```python
from build123d import *

# Parameters (mm, degrees)
BOSS_EXTRUDE3_DEPTH = 23
SKETCH5_W           = 86
SKETCH5_H           = 89
BOSS_EXTRUDE4_DEPTH = 4
SKETCH7_W           = 86
SKETCH7_H           = 4
CUT_EXTRUDE2_DEPTH  = 6
FILLET2_R           = 2
FILLET3_R           = 2
SKETCH8_R           = 1.6
BOSS_EXTRUDE5_DEPTH = 4
FILLET4_R           = 2


# Some blends are built 0.0001 mm under size
with BuildPart() as part:
    # Sketch2 → Boss-Extrude3 (new body)
    with BuildSketch(Plane(origin=(0, 0, 0), x_dir=(1, 0, 0), z_dir=(0, 1, 0))):
        Polygon((-45.956172868, 28.642659602), (-45.956172868, -110.357340398), (40.043827132, -110.357340398), (40.043827132, 28.642659602), (36.043827132, 28.642659602), (36.043827132, -106.357340398), (-41.956172868, -106.357340398), (-41.956172868, 28.642659602), align=None)
    extrude(amount=BOSS_EXTRUDE3_DEPTH)

    # Sketch5 → Boss-Extrude4 (add)
    with BuildSketch(Plane.XZ):
        with Locations((-2.956172868, 65.857340398)):
            Rectangle(SKETCH5_W, SKETCH5_H)
    extrude(amount=BOSS_EXTRUDE4_DEPTH)

    # Sketch7 → Cut-Extrude2 (cut)
    with BuildSketch(Plane.XZ):
        with Locations((-2.956172868, -20.642659602)):
            Rectangle(SKETCH7_W, SKETCH7_H)
    extrude(amount=-CUT_EXTRUDE2_DEPTH, mode=Mode.SUBTRACT)

    # Fillet2
    fillet2_edges = [part.edges().sort_by_distance(p)[0] for p in [
        (40.043827132, -4, 65.857340398),
        (-2.956172868, -4, 110.357340398),
        (-45.956172868, -4, 65.857340398),
    ]]
    fillet(fillet2_edges, radius=FILLET2_R)

    # Fillet3
    # the kernel refuses this fillet: 2 mm, written as the material it takes off along each edge
    with BuildSketch(Plane(origin=(38.043827132, -2, 108.357340398), x_dir=(1, 0, 0), z_dir=(0, 0, 1))) as fillet3_piece_1_section:
        Polygon((0, 0), (FILLET3_R, 0), (FILLET3_R, -FILLET3_R), (0, -FILLET3_R), align=None)
    fillet3_piece_1 = extrude(amount=FILLET3_R, mode=Mode.PRIVATE)
    fillet3_piece_1 = fillet3_piece_1 - Plane(origin=(38.043827132, -2, 108.357340398), x_dir=(-0.7071067811865475, 0.7071067811865475, 0), z_dir=(0, 0, 1)) * Sphere(FILLET3_R, mode=Mode.PRIVATE)
    add(fillet3_piece_1, mode=Mode.SUBTRACT)
    with BuildSketch(Plane(origin=(-43.956172868, -2, 108.357340398), x_dir=(0, 0, 1), z_dir=(-1, 0, 0))) as fillet3_piece_2_section:
        Polygon((0, 0), (FILLET3_R, 0), (FILLET3_R, -FILLET3_R), (0, -FILLET3_R), align=None)
    fillet3_piece_2 = extrude(amount=FILLET3_R, mode=Mode.PRIVATE)
    fillet3_piece_2 = fillet3_piece_2 - Plane(origin=(-43.956172868, -2, 108.357340398), x_dir=(0, 0.7071067811865475, -0.7071067811865475), z_dir=(-1, 0, 0)) * Sphere(FILLET3_R, mode=Mode.PRIVATE)
    add(fillet3_piece_2, mode=Mode.SUBTRACT)
    with BuildSketch(Plane(origin=(-41.956172868, -5, -28.642659602), x_dir=(-1, 0, 0), z_dir=(0, 1, 0)), Plane(origin=(-45.956172868, -5, -28.642659602), x_dir=(0, 0, 1), z_dir=(0, 1, 0))) as fillet3_piece_3:
        with BuildLine():
            CenterArc((FILLET3_R, FILLET3_R), FILLET3_R, 180, 90)
            Line((0, FILLET3_R), (0, 0))
            Line((0, 0), (FILLET3_R, 0))
        make_face()
    extrude(amount=33, mode=Mode.SUBTRACT)
    with BuildSketch(Plane(origin=(40.043827132, -2, 110.357340398), x_dir=(-1, 0, 0), z_dir=(0, 1, 0)), Plane(origin=(-45.956172868, -2, 110.357340398), x_dir=(0, 0, -1), z_dir=(0, 1, 0))) as fillet3_piece_4:
        with BuildLine():
            CenterArc((FILLET3_R, -FILLET3_R), FILLET3_R, 90, 90)
            Line((0, -FILLET3_R), (0, 0))
            Line((0, 0), (FILLET3_R, 0))
        make_face()
    extrude(amount=30, mode=Mode.SUBTRACT)

    # Sketch8 → Boss-Extrude5 (add)
    # profile 1 of 4: a face of its own
    with BuildSketch(Plane(origin=(0, 23, 0), x_dir=(1, 0, 0), z_dir=(0, 1, 0))):
        with BuildLine():
            Line((40.043827132, -95.857340398), (40.043827132, -86.857340398))
            Line((40.043827132, -86.857340398), (44.543827132, -86.857340398))
            ThreePointArc((44.543827132, -86.857340398), (49.043827132, -91.357340398), (44.543827132, -95.857340398))
            Line((44.543827132, -95.857340398), (40.043827132, -95.857340398))
        make_face()
        with Locations(Location((44.543827132, -91.357340398, 0), (0, 0, 270))):
            Circle(SKETCH8_R, mode=Mode.SUBTRACT)
    # profile 2 of 4: a face of its own
    with BuildSketch(Plane(origin=(0, 23, 0), x_dir=(1, 0, 0), z_dir=(0, 1, 0))):
        with BuildLine():
            Line((-50.456172868, 13.142659602), (-45.956172868, 13.142659602))
            Line((-45.956172868, 13.142659602), (-45.956172868, 4.142659602))
            Line((-45.956172868, 4.142659602), (-50.456172868, 4.142659602))
            ThreePointArc((-50.456172868, 4.142659602), (-54.956172868, 8.642659602), (-50.456172868, 13.142659602))
        make_face()
        with Locations(Location((-50.456172868, 8.642659602, 0), (0, 0, 270))):
            Circle(SKETCH8_R, mode=Mode.SUBTRACT)
    # profile 3 of 4: a face of its own
    with BuildSketch(Plane(origin=(0, 23, 0), x_dir=(1, 0, 0), z_dir=(0, 1, 0))):
        with BuildLine():
            Line((44.543827132, 13.142659602), (40.043827132, 13.142659602))
            Line((40.043827132, 13.142659602), (40.043827132, 4.142659602))
            Line((40.043827132, 4.142659602), (44.543827132, 4.142659602))
            ThreePointArc((44.543827132, 4.142659602), (49.043827132, 8.642659602), (44.543827132, 13.142659602))
        make_face()
        with Locations(Location((44.543827132, 8.642659602, 0), (0, 0, 270))):
            Circle(SKETCH8_R, mode=Mode.SUBTRACT)
    # profile 4 of 4: a face of its own
    with BuildSketch(Plane(origin=(0, 23, 0), x_dir=(1, 0, 0), z_dir=(0, 1, 0))):
        with BuildLine():
            Line((-50.456172868, -86.857340398), (-45.956172868, -86.857340398))
            Line((-45.956172868, -86.857340398), (-45.956172868, -95.857340398))
            Line((-45.956172868, -95.857340398), (-50.456172868, -95.857340398))
            ThreePointArc((-50.456172868, -95.857340398), (-54.956172868, -91.357340398), (-50.456172868, -86.857340398))
        make_face()
        with Locations(Location((-50.456172868, -91.357340398, 0), (0, 0, 270))):
            Circle(SKETCH8_R, mode=Mode.SUBTRACT)
    extrude(amount=-BOSS_EXTRUDE5_DEPTH)

    # Fillet4
    fillet4_edges = [part.edges().sort_by_distance(p)[0] for p in [
        (40.043827132, 11.5, -28.642659602),
        (36.043827132, 11.5, -28.642659602),
    ]]
    fillet(fillet4_edges, radius=FILLET4_R - 0.0001)  # a hair under: the kernel refuses the full size


solid = part.part
```
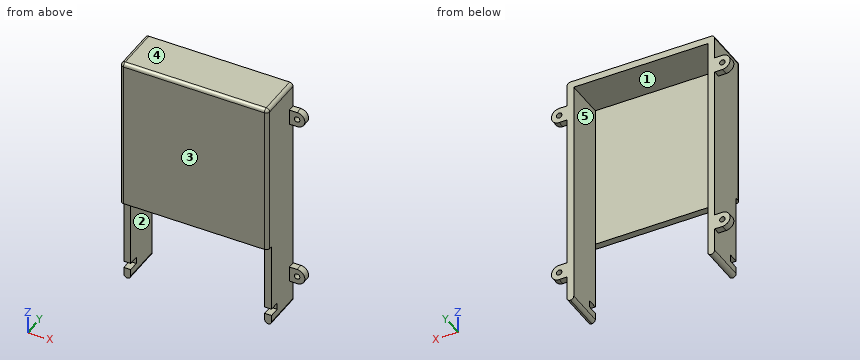
Geometry check sheet. Reference: the model listing, model coordinates, mm. Face numbers are marked on the shaded views. A direction names the side the tool comes from. Coordinates: 2 decimals unless noted, no trailing zeros. Loops run counter-clockwise (first coordinate to the right, second up) from the corner with the lowest first, then second, coordinate; pieces in that order, holes last. Notation, with made-up numbers: (72.5, -21.5) - (84.5, -21.5) arc R16 ccw to (84.5, -14.5) - close; hole circle Ø9 at (-3, 86.25). An arc over 180 degrees is marked (long way). One line per item, written item: value. Start each with the question number.
(1) Mould release check, pull along X, two halves, no side actions. Record for the marked faces 1, 2 and 3: released by +X, released by -X, zero draft, split by the parting line, or undercut.
(2) Depth check by flat-ended pin: P1, Ø2, axis at x = -43, z = 4, coming from the -Y side; P2, Ø4, axis at y = 19.5, z = 14.5, coming from the +X side; P3, Ø2, axis at x = 36.5, y = 6, coming from the -Z side; P4, Ø1.9, axis at x = 44.54, z = 91.36, coming from the +Y side. Enter the tip coordinate at first touch or a pass-through.
(3) Cross-section at A-A on z = -15. Enter the section's corners in (x, y).
(4) Cross-section at D-D on x = -38. Enter the section's corners in (y, z), plus the area to 3 significant figures.
(5) Cross-section at C-C on z = 77.5. Enter the section's corners in (x, y), plus the area to 3 significant figures.
(6) Material ranges on line 1 (X direction, y = 12, z = 87); line 2 (X direction, y = 19.5, z = -7.5); line 3 (Z direction, x = -39, y = -0.5), recorded low to high. Write a range as [from, to].
(7) Tool access check on the marked faces 4 and 5. Record the directions out of +Z, -Z, +X, -X, +Y, -Y that give a thin tool (end or side, any length) a straight path to the whole face; none if there is none.
(8) Cross-section at B-B on y = 2.5. Count the separate pieces of the cut face and the enclosed holes in it, plus the area to 3 significant figures.
Results below:
1. face 1: undercut
1. face 2: undercut
1. face 3: zero draft
2. P1: stops at y = 0
2. P2: stops at x = 40.04
2. P3: stops at z = -28.57
2. P4: passes through
3. outline: (-45.96, 0) - (-41.96, 0) - (-41.96, 23) - (-45.96, 23) - close; (36.04, 0) - (40.04, 0) - (40.04, 23) - (36.04, 23) - close
4. outline: (-4, 21.36) - (0, 21.36) - (0, 106.36) - (23, 106.36) - (23, 110.36) - (-2, 110.36) arc R2 ccw to (-4, 108.36) - close
4. area: 447 mm2
5. outline: (-45.96, -2) arc R2 ccw to (-43.96, -4) - (38.04, -4) arc R2 ccw to (40.04, -2) - (40.04, 23) - (36.04, 23) - (36.04, 0) - (-41.96, 0) - (-41.96, 23) - (-45.96, 23) - close
5. area: 526 mm2
6. line 1: x = [-45.96, -41.96], [36.04, 40.04]
6. line 2: x = [-54.81, -51.58], [-49.34, -41.96], [36.04, 43.42], [45.66, 48.9]
6. line 3: z = [21.36, 110.36]
7. face 4: +Z, +X, -X, +Y, -Y
7. face 5: -Z, +Y
8. separate pieces: 3
8. enclosed holes: 0
8. area: 1,390 mm2
